Geometry check sheet. Reference: the model listing, model coordinates, mm. Face numbers are marked on the shaded views. Round coordinates to 2 decimals unless told otherwise and drop trailing zeros. Loops run counter-clockwise (first coordinate to the right, second up) from the corner with the lowest first, then second, coordinate; pieces in that order, holes last. Notation, with made-up numbers: (50, 37) -> (94, 37) arc R22 cw to (94, 44) -> close; hole circle Ø8 at (75, 59.25). An arc over 180 degrees is marked (long way). Use one line per item in the form item = value.
from build123d import *

# Parameters (mm, degrees)
SKETCH_1_W          = 15
SKETCH_1_H          = 15
SKETCH_1_W_2        = 12
SKETCH_1_H_2        = 12
EXTRUDE_1_DEPTH     = 345
SKETCH_2_R          = 2
CUT_EXTRUDE_1_DEPTH = 346.40736819
SKETCH_3_R          = 2
CUT_EXTRUDE_2_DEPTH = 346.40736819


with BuildPart() as part:
    # ｽｹｯﾁ1 → 押し出し-薄板1 (new body)
    with BuildSketch(Plane(origin=(0, 0, 0), x_dir=(1, 0, 0), z_dir=(0, 1, 0))):
        Rectangle(SKETCH_1_W, SKETCH_1_H)
        Rectangle(SKETCH_1_W_2, SKETCH_1_H_2, mode=Mode.SUBTRACT)
    extrude(amount=EXTRUDE_1_DEPTH)

    # ｽｹｯﾁ2 → ｶｯﾄ - 押し出し1 (cut, through all)
    with BuildSketch(Plane(origin=(7.5, 0, 0), x_dir=(0, 0, -1), z_dir=(1, 0, 0))):
        with Locations((0, 5)):
            Circle(SKETCH_2_R)
        with Locations((0, 297.5)):
            Circle(SKETCH_2_R)
        with Locations((0, 337.5)):
            Circle(SKETCH_2_R)
        with Locations((0, 327.5)):
            Circle(SKETCH_2_R)
    extrude(amount=-CUT_EXTRUDE_1_DEPTH, mode=Mode.SUBTRACT)

    # ｽｹｯﾁ3 → ｶｯﾄ - 押し出し2 (cut, through all)
    with BuildSketch(Plane.XY.offset(7.5)):
        with Locations((0, 225)):
            Circle(SKETCH_3_R)
        with Locations((0, 215)):
            Circle(SKETCH_3_R)
    extrude(amount=-CUT_EXTRUDE_2_DEPTH, mode=Mode.SUBTRACT)


solid = part.part
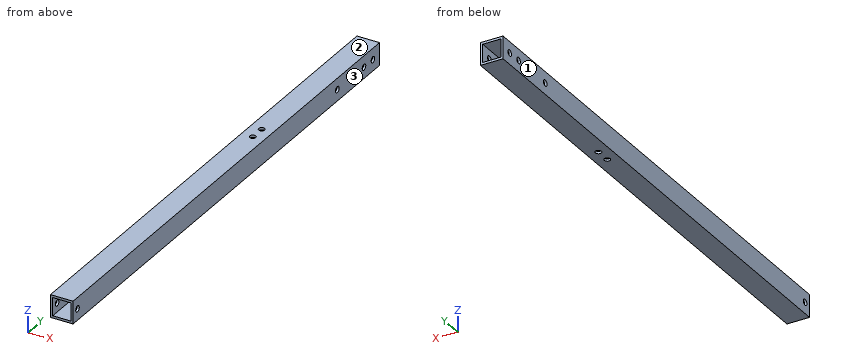
1. Section check A-A (y = 79). Record the boundary of the cut face in (x, z), then the cut area to 3 significant figures.
Return value:
outline = (-7.5, -7.5) -> (7.5, -7.5) -> (7.5, 7.5) -> (-7.5, 7.5) -> close; hole (-6, -6) -> (6, -6) -> (6, 6) -> (-6, 6) -> close
area = 81.0 mm2
2. Material ranges on line 1 along Y through (x, z) = (-7.1, 0); line 2 along Y through (x, z) = (6.75, 0.5); line 3 along Y through (x, z) = (0, -6.8), recorded low to high.
Return value:
line_1 = 0 to 3, 7 to 295.5, 299.5 to 325.5, 329.5 to 335.5, 339.5 to 345
line_2 = 0 to 3.06, 6.94 to 295.56, 299.44 to 325.56, 329.44 to 335.56, 339.44 to 345
line_3 = 0 to 213, 217 to 223, 227 to 345
3. Mould release check, pull along X, two halves, no side actions. Record for the marked faces 1, 2 and 3: released by +X, released by -X, zero draft, split by the parting line, or undercut.
Return value:
face_1 = released by -X
face_2 = zero draft
face_3 = released by +X
